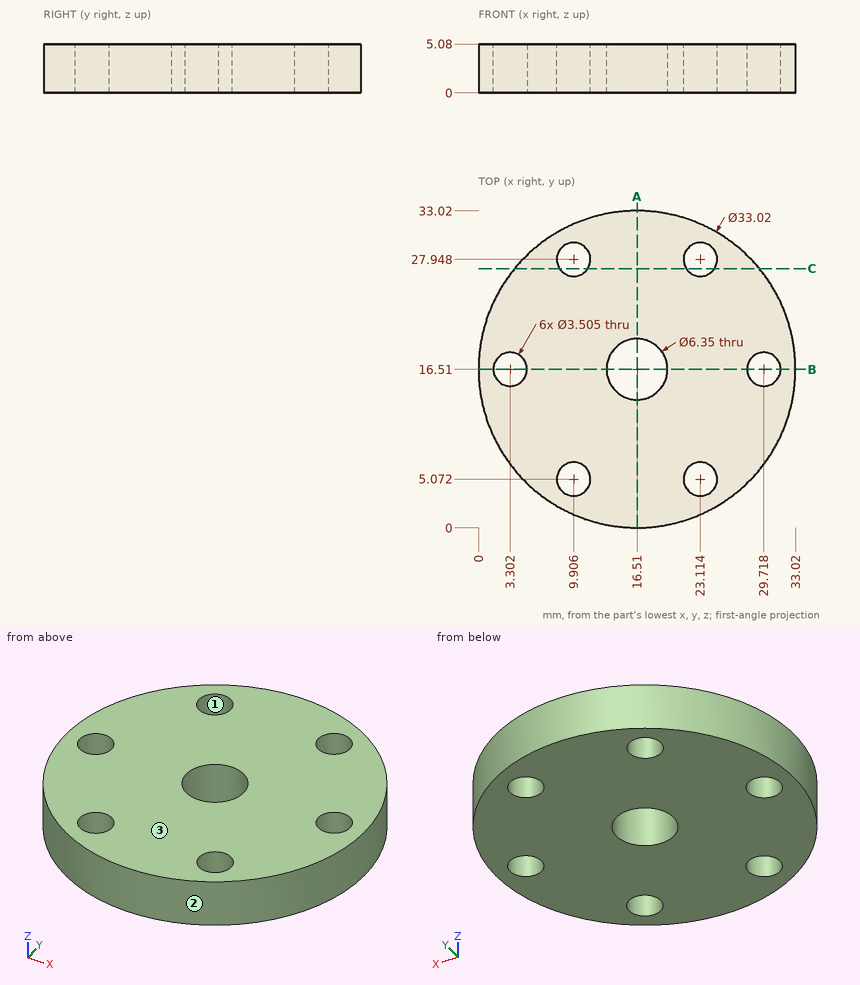
Geometry check sheet. Reference: drawing and pictorial views, mm from the part's lowest x, y, z. Round coordinates to 2 decimals unless told otherwise and drop trailing zeros. Write each loop counter-clockwise with the first axis right and the second up, starting at its lowest first coordinate (ties: lowest second). Pieces come first, ordered by that corner, then holes. Notation, with made-up numbers: (47, -35.5) -> (66, -35.5) arc R12 cw to (66, -21.5) -> close; hole circle Ø2 at (-29, 46.5). An arc over 180 degrees is marked (long way). One line per question, with ' | ' between items. Start each with the question number.
1. Scan lines: line 1 along Y through (x, z) = (16.51, 2.85) (1 decimal); line 2 along X through (y, z) = (28, 3.5) (1 decimal); line 3 along X through (y, z) = (6, 1.8) (1 decimal). Record each from-to range of solid material in increasing order. Write a range as from..to.
2. Release check for a two-part mould opening along X. For the marked faces 1, 2 and 3 record: +X half, -X half, draft (parallel to the pull), parting line (faces both ways), or undercut.
3. Sectioned sample at A-A, the plane x = 16.51. Record the cut outline in (y, z) (1 decimal).
4. Sectioned sample at C-C, the plane y = 27. Record the cut outline in (x, z).
5. Sectioned sample at B-B, the plane y = 16.51. Count the separate pieces of the cut face and the enclosed holes in it.
6. Depth check by flat-ended pin: pin 1 (1.5 mm diameter, centred on x = 24.5, z = 1.5, fed in from +Y); pin 2 (2 mm diameter, centred on y = 19.5, z = 1.5, fed in from -X); pin 3 (3 mm diameter, centred on x = 29.718, y = 16.51, fed in from +Z); pin 4 (1.5 mm diameter, centred on y = 17.5, z = 2.5, fed in from +X). Enter the tip coordinate at first touch or a pass-through.
Taken from the geometry:
1) line 1: y = 0..13.3, 19.7..33 | line 2: x = 4.7..8.2, 11.7..21.4, 24.9..28.4 | line 3: x = 3.8..8.4, 11.4..21.6, 24.6..29.2
2) face 1: undercut | face 2: parting line | face 3: draft
3) outline: (0, 0) -> (13.3, 0) -> (13.3, 5.1) -> (0, 5.1) -> close; (19.7, 0) -> (33, 0) -> (33, 5.1) -> (19.7, 5.1) -> close
4) outline: (3.76, 0) -> (8.43, 0) -> (8.43, 5.08) -> (3.76, 5.08) -> close; (11.38, 0) -> (21.64, 0) -> (21.64, 5.08) -> (11.38, 5.08) -> close; (24.59, 0) -> (29.26, 0) -> (29.26, 5.08) -> (24.59, 5.08) -> close
5) separate pieces: 4 | enclosed holes: 0
6) pin 1: stops at y = 31.35 | pin 2: stops at x = 0.12 | pin 3: passes through | pin 4: stops at x = 33.02
